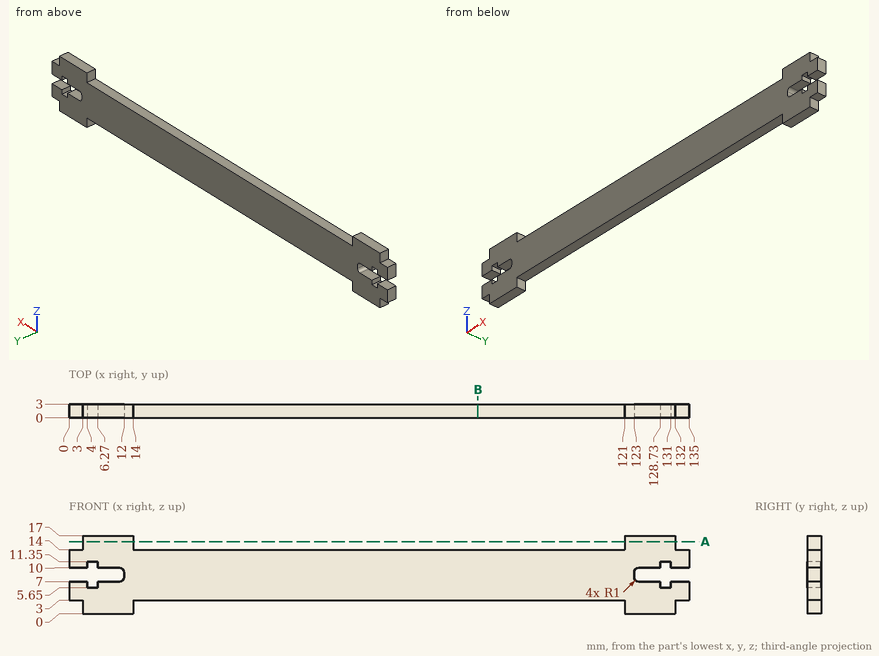
Can you work these out from the drawing? Everything is in mm from the part's minimum corner. Coordinates: 2 decimals unless noted, no trailing zeros. Order: outer loops, then holes, each group sorted by start corner. A loop starts at its lowest first (then second) coordinate and runs counter-clockwise, first axis right, second up. Notation, with made-up numbers: M 36.5,-19 L 65.5,-19 A17 ccw 65.5,6 Z; hole C 9,58.25 d7. An arc over 180 degrees is marked long. Answer as CSV lines item,"result". Start each with the question number.
1. I want a section at B-B, the plane x = 89. Write out the boundary of the cut face in (y, z).
2. For pin 1 (0.9 mm diameter, centred on x = 133.5, y = 1, fed in from -Z); pin 2 (3 mm diameter, centred on x = 91, z = 12, fed in from -Y); pin 3 (0.9 mm diameter, centred on x = 132.5, y = 2, fed in from +Z), each with a flat end and sliding along its axis, tell me the tip position at first contact or that it passes through.
3. I need wall thicknesses on line 1 (X direction, y = 2.5, z = 10.5); line 2 (Z direction, x = 127, y = 0.5); line 3 (Z direction, x = 74.5, y = 1.25). Which ranges of each line are inside material? Lowest first, please. Write a range as [from, to].
4. I want a section at A-A, the plane z = 15.75. Write out the boundary of the cut face in (x, y).
Recorded:
1,outline,"M 0,3 L 3,3 L 3,14 L 0,14 Z"
2,pin 1,"stops at z = 3"
2,pin 2,"stops at y = 0"
2,pin 3,"stops at z = 14"
3,line 1,"x = [0, 4], [6.27, 128.73], [131, 135]"
3,line 2,"z = [0, 7], [10, 17]"
3,line 3,"z = [3, 14]"
4,outline,"M 3,0 L 14,0 L 14,3 L 3,3 Z; M 121,0 L 132,0 L 132,3 L 121,3 Z"
